```python
from build123d import *

# Parameters (mm, degrees)
SKETCH1_R               = 7.55
SKETCH1_R_2             = 5.15
BOSS_EXTRUDE1_DEPTH     = 12
SKETCH2_R               = 11.1
CUT_EXTRUDE1_DEPTH      = 9
SKETCH3_R               = 1.65
CUT_EXTRUDE2_DEPTH      = 52.971145841
CUT_EXTRUDE3_DEPTH      = 6
CUT_EXTRUDE4_DEPTH      = 48.634021455
CUT_EXTRUDE4_DEPTH_BACK = 48.634021455
SKETCH5_W               = 10
SKETCH5_H               = 10
CHAMFER1_SIZE           = 2
CHAMFER2_SIZE           = 0.5
SKETCH7_R               = 2.6
CUT_EXTRUDE6_DEPTH      = 33
CUT_EXTRUDE7_DEPTH      = 48.634021455
CUT_EXTRUDE7_DEPTH_BACK = 48.634021455
SKETCH8_W               = 5
SKETCH8_H               = 8
CHAMFER3_SIZE           = 1
CHAMFER4_SIZE           = 0.6
SKETCH9_W               = 2
SKETCH9_H               = 4.3
CUT_EXTRUDE8_DEPTH      = 8


with BuildPart() as part:
    # Sketch1 → Boss-Extrude1 (new, symmetric)
    with BuildSketch(Plane.XY):
        with BuildLine():
            Line((27, -30), (-27, -30))
            ThreePointArc((-27, -30), (-32.656854249, -27.656854249), (-35, -22))
            Line((-35, -22), (-35, 22))
            ThreePointArc((-35, 22), (-32.656854249, 27.656854249), (-27, 30))
            Line((-27, 30), (27, 30))
            ThreePointArc((27, 30), (32.656854249, 27.656854249), (35, 22))
            Line((35, 22), (35, -22))
            ThreePointArc((35, -22), (32.656854249, -27.656854249), (27, -30))
        make_face()
        with Locations((-20, 15)):
            Circle(SKETCH1_R, mode=Mode.SUBTRACT)
        with Locations((20, 15)):
            Circle(SKETCH1_R, mode=Mode.SUBTRACT)
        with Locations((20, -15)):
            Circle(SKETCH1_R_2, mode=Mode.SUBTRACT)
        with Locations((-20, -15)):
            Circle(SKETCH1_R_2, mode=Mode.SUBTRACT)
    extrude(amount=BOSS_EXTRUDE1_DEPTH, both=True)

    # Sketch2 → Cut-Extrude1 (cut)
    with BuildSketch(Plane.XY.offset(12)):
        with Locations((-20, -15)):
            Circle(SKETCH2_R)
    extrude(amount=-CUT_EXTRUDE1_DEPTH, mode=Mode.SUBTRACT)

    # Sketch3 → Cut-Extrude2 (cut, through all)
    with BuildSketch(Plane.XY.offset(12)):
        with Locations((-25.656854249, -9.343145751)):
            Circle(SKETCH3_R)
        with Locations((-14.343145751, -9.343145751)):
            Circle(SKETCH3_R)
        with Locations((-14.343145751, -20.656854249)):
            Circle(SKETCH3_R)
        with Locations((-25.656854249, -20.656854249)):
            Circle(SKETCH3_R)
    extrude(amount=-CUT_EXTRUDE2_DEPTH, mode=Mode.SUBTRACT)

    # Sketch4 → Cut-Extrude3 (cut)
    with BuildSketch(Plane(origin=(0, 0, -12), x_dir=(-1, 0, 0), z_dir=(0, 0, -1))):
        Polygon((17.29883669, -10.135120751), (16.50686169, -7.179429811), (13.55117075, -6.387454811), (11.387454811, -8.55117075), (12.179429811, -11.50686169), (15.135120751, -12.29883669), align=None)
        Polygon((23.49313831, -7.179429811), (22.70116331, -10.135120751), (24.864879249, -12.29883669), (27.820570189, -11.50686169), (28.612545189, -8.55117075), (26.44882925, -6.387454811), align=None)
        Polygon((24.864879249, -17.70116331), (22.70116331, -19.864879249), (23.49313831, -22.820570189), (26.44882925, -23.612545189), (28.612545189, -21.44882925), (27.820570189, -18.49313831), align=None)
        Polygon((15.135120751, -17.70116331), (12.179429811, -18.49313831), (11.387454811, -21.44882925), (13.55117075, -23.612545189), (16.50686169, -22.820570189), (17.29883669, -19.864879249), align=None)
    extrude(amount=-CUT_EXTRUDE3_DEPTH, mode=Mode.SUBTRACT)

    # Sketch5 → Cut-Extrude4 (cut, two sides: drawn at the far end of the back side and taken through both)
    with BuildSketch(Plane(origin=(0, 0, 0), x_dir=(1, 0, 0), z_dir=(0, 1, 0)).offset(-CUT_EXTRUDE4_DEPTH_BACK)):
        Rectangle(SKETCH5_W, SKETCH5_H)
    extrude(amount=CUT_EXTRUDE4_DEPTH + CUT_EXTRUDE4_DEPTH_BACK, mode=Mode.SUBTRACT)

    # Chamfer1
    chamfer1_edges = [part.edges().sort_by_distance(p)[0] for p in [
        (35, 0, -12),
        (32.656854249, -27.656854249, -12),
        (0, -30, -12),
        (-32.656854249, -27.656854249, -12),
        (32.656854249, -27.656854249, 12),
        (35, 0, 12),
        (32.656854249, 27.656854249, 12),
        (0, 30, 12),
        (-32.656854249, 27.656854249, 12),
        (-35, 0, 12),
        (-32.656854249, -27.656854249, 12),
        (-35, 0, -12),
        (0, -30, 12),
        (-32.656854249, 27.656854249, -12),
        (0, 30, -12),
        (32.656854249, 27.656854249, -12),
    ]]
    chamfer(chamfer1_edges, length=CHAMFER1_SIZE)

    # Chamfer2
    chamfer2_edges = [part.edges().sort_by_distance(p)[0] for p in [
        (-27.55, 15, -12),
        (-27.55, 15, 12),
        (12.45, 15, -12),
        (12.45, 15, 12),
        (14.85, -15, -12),
        (14.85, -15, 12),
        (-31.1, -15, 12),
    ]]
    chamfer(chamfer2_edges, length=CHAMFER2_SIZE)

    # Sketch7 → Cut-Extrude6 (cut)
    with BuildSketch(Plane(origin=(35, 0, 0), x_dir=(0, 0, -1), z_dir=(1, 0, 0))):
        with Locations((0, -2)):
            Circle(SKETCH7_R)
    extrude(amount=-CUT_EXTRUDE6_DEPTH, mode=Mode.SUBTRACT)

    # Sketch8 → Cut-Extrude7 (cut, two sides: drawn at the far end of the back side and taken through both)
    with BuildSketch(Plane.XY.offset(-CUT_EXTRUDE7_DEPTH_BACK)):
        with Locations((14.5, -2)):
            Rectangle(SKETCH8_W, SKETCH8_H)
    extrude(amount=CUT_EXTRUDE7_DEPTH + CUT_EXTRUDE7_DEPTH_BACK, mode=Mode.SUBTRACT)

    # Chamfer3
    chamfer3_edges = [part.edges().sort_by_distance(p)[0] for p in [
        (35, -2, 2.6),
    ]]
    chamfer(chamfer3_edges, length=CHAMFER3_SIZE)

    # Chamfer4
    chamfer4_edges = [part.edges().sort_by_distance(p)[0] for p in [
        (-5, -30, 0),
        (0, -30, -5),
        (5, -30, 0),
        (0, -30, 5),
        (-5, 30, 0),
        (0, 30, 5),
        (5, 30, 0),
        (0, 30, -5),
    ]]
    chamfer(chamfer4_edges, length=CHAMFER4_SIZE)

    # Sketch9 → Cut-Extrude8 (cut)
    with BuildSketch(Plane.XZ.offset(30)):
        with Locations((19, -7)):
            Rectangle(SKETCH9_W, SKETCH9_H)
    extrude(amount=-CUT_EXTRUDE8_DEPTH, mode=Mode.SUBTRACT)


solid = part.part
```
Input: part model. Units: mm. Frame: model coordinates. A direction names the side the tool comes from. Give positions to 0.01 mm unless a question says otherwise; leave off trailing zeros. Order: outer loops, then holes, each group sorted by start corner. A loop starts at its lowest first (then second) coordinate and runs counter-clockwise, first axis right, second up. Notation, with made-up numbers: M -28,35.25 L 22,35.25 A16 cw 22,50.25 Z; hole C -35.5,-11.5 d4. An arc over 180 degrees is marked long. Return JSON: item names as keys, results as strings.
Item 1: Cut plane A-A (y = 15). Return loops of the section in (x, z), then the cut area to 3 significant figures.
Solutions:
{"outline": "M -35,-10 L -33,-12 L -28.05,-12 L -27.55,-11.5 L -27.55,11.5 L -28.05,12 L -33,12 L -35,10 Z; M -12.45,-11.5 L -11.95,-12 L 11.95,-12 L 12.45,-11.5 L 12.45,11.5 L 11.95,12 L -11.95,12 L -12.45,11.5 Z; M 27.55,-11.5 L 28.05,-12 L 33,-12 L 35,-10 L 35,10 L 33,12 L 28.05,12 L 27.55,11.5 Z; hole M -5,-5 L 5,-5 L 5,5 L -5,5 Z", "area": "846 mm^2"}
Item 2: Pull-direction query (X, two-part tool) for faces 1 (the flat face through (34, 0, 11)), 2 (the flat face through (-28.22, -19.99, -9.04)), 3 (the flat face through (-6, 30, 0)); classes: +X half, -X half, draft (parallel to the pull), parting line (faces both ways), or undercut.
Solutions:
{"face 1": "+X half", "face 2": "undercut", "face 3": "draft"}
Item 3: Access query for faces 4 (the flat face through (19, -22, -7)), 5 (the flat face through (35, 0, 5)), 6 (the flat face through (-23.1, -8.64, -9.04)). Directions: +Z, -Z, +X, -X, +Y, -Y. A direction counts if a zero-diameter tool reaches every point of the face in a straight line with its end or side. Return the directions, or none.
Solutions:
{"face 4": "-Y", "face 5": "+Z, -Z, +X, +Y, -Y", "face 6": "-Z"}
Item 4: Cut plane D-D (y = -2). Return loops of the section in (x, z).
Solutions:
{"outline": "M -35,-10 L -33,-12 L 12,-12 L 12,-2.6 L 5,-2.6 L 5,-5 L -5,-5 L -5,5 L 5,5 L 5,2.6 L 12,2.6 L 12,12 L -33,12 L -35,10 Z; M 17,-12 L 33,-12 L 35,-10 L 35,-3.6 L 34,-2.6 L 17,-2.6 Z; M 17,2.6 L 34,2.6 L 35,3.6 L 35,10 L 33,12 L 17,12 Z"}
Item 5: Cut plane C-C (x = -4). Return loops of the section in (y, z), then the cut area to 3 significant figures.
Solutions:
{"outline": "M -30,-10 L -28,-12 L 28,-12 L 30,-10 L 30,-5.6 L 29.4,-5 L -29.4,-5 L -30,-5.6 Z; M -30,5.6 L -29.4,5 L 29.4,5 L 30,5.6 L 30,10 L 28,12 L -28,12 L -30,10 Z", "area": "831 mm^2"}
Item 6: First-contact query: P1, Ø1.3, axis at y = -26.5, z = -8, coming from the +X side. Flat tip, straight axial feed; report the tip coordinate or a pass-through.
Solutions:
{"P1": "x = 34.01"}
Item 7: Ray query, probe 1 along Y at (x, z) = (-20, -5.5); probe 2 along X at (y, z) = (15.5, 3.5); probe 3 along X at (y, z) = (2.5, -3.75). Return the intervals inside material, ascending.
Solutions:
{"probe 1": "-30 to -20.15, -9.85 to 7.45, 22.55 to 30", "probe 2": "-35 to -27.53, -12.47 to -5, 5 to 12.47, 27.53 to 35", "probe 3": "-35 to -5, 5 to 35"}
Item 8: Cut plane B-B (x = -20). Return loops of the section in (y, z).
Solutions:
{"outline": "M -30,-10 L -28,-12 L -20.15,-12 L -20.15,3 L -26.1,3 L -26.1,11.5 L -26.6,12 L -28,12 L -30,10 Z; M -9.85,-12 L 6.95,-12 L 7.45,-11.5 L 7.45,11.5 L 6.95,12 L -3.4,12 L -3.9,11.5 L -3.9,3 L -9.85,3 Z; M 22.55,-11.5 L 23.05,-12 L 28,-12 L 30,-10 L 30,10 L 28,12 L 23.05,12 L 22.55,11.5 Z"}
